Input: part model. Units: mm. Frame: model coordinates. Face numbers are marked on the shaded views. A direction names the side the tool comes from. Round coordinates to 2 decimals unless told otherwise and drop trailing zeros. Loops run counter-clockwise (first coordinate to the right, second up) from the corner with the lowest first, then second, coordinate; pieces in that order, holes last. Notation, with made-up numbers: M 35,39.25 L 94,39.25 A18 cw 94,69.25 Z; hole C -26,-19 d2. An arc over 180 degrees is marked long. Return JSON: item names as keys, results as strings. Group by question number.
1) Section D-D (y = 0.5). Output: boundary loops of the cut face in (x, z).
2) Contact query for flat-ended pins moving along their axis: P1, Ø23.5, axis at x = 0, y = 0.5, coming from the +Z side; P2, Ø14.5, axis at x = -9.5, z = 19, coming from the +Y side; P3, Ø2, axis at x = -23.5, y = -11.5, coming from the +Z side. Output: stop coordinate, or through.
3) Section A-A (z = 35). Output: boundary loops of the cut face in (x, y).
4) Material intervals for line 1 (X direction, y = -15, z = 1); line 2 (Y direction, x = 15.5, z = 1.9); line 3 (Y direction, x = 15, z = 1), sorted ascending. Write a range as from..to.
5) Section B-B (y = 16). Output: boundary loops of the cut face in (x, z), plus the area to 3 significant figures.
6) Section C-C (x = -15.5). Output: boundary loops of the cut face in (y, z).
7) Access query for the marked faces 1 and 2. Directions: +Z, -Z, +X, -X, +Y, -Y. A direction counts if a zero-diameter tool reaches every point of the face in a straight line with its end or side. Return the directions, or none.
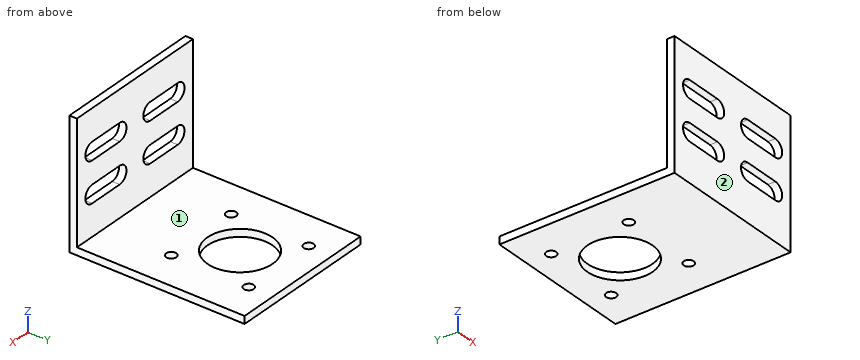
from build123d import *

# Parameters (mm, degrees)
SKETCH_1_W               = 60
SKETCH_1_H               = 70
SKETCH_1_R               = 13
EXTRUDE_1_DEPTH          = 3
SKETCH_2_W               = 60
SKETCH_2_H               = 51
EXTRUDE_2_DEPTH          = 3
SKETCH_3_R               = 2
CUT_EXTRUDE_1_DEPTH      = 10
MIRROR_3_COPY_1_SKETCH_R = 2
MIRROR_3_COPY_1_DEPTH    = 10
CUT_EXTRUDE_2_DEPTH      = 10
MIRROR_5_COPY_1_DEPTH    = 10


with BuildPart() as part:
    # 草图1 → 凸台-拉伸1 (new body)
    with BuildSketch(Plane.XY):
        with Locations((0, -9.5)):
            Rectangle(SKETCH_1_W, SKETCH_1_H)
        with Locations((0, 0.5)):
            Circle(SKETCH_1_R, mode=Mode.SUBTRACT)
    extrude(amount=EXTRUDE_1_DEPTH)

    # 草图2 → 凸台-拉伸2 (add)
    with BuildSketch(Plane.XZ.offset(44.5)):
        with Locations((0, 25.5)):
            Rectangle(SKETCH_2_W, SKETCH_2_H)
    extrude(amount=-EXTRUDE_2_DEPTH)

    # 草图3 → 切除-拉伸1 (cut)
    with BuildSketch(Plane.XY.offset(3)):
        with Locations((-15.5, 16)):
            Circle(SKETCH_3_R)
    cut_extrude_1 = extrude(amount=-CUT_EXTRUDE_1_DEPTH, mode=Mode.SUBTRACT)

    # 镜向1: 切除-拉伸1 across plane
    add(cut_extrude_1.mirror(Plane(origin=(0, 0, 0), x_dir=(0, 0, 1), z_dir=(1, 0, 0))), mode=Mode.SUBTRACT)

    # 镜向3: 切除-拉伸1 across plane
    add(cut_extrude_1.mirror(Plane.ZX.offset(0.5)), mode=Mode.SUBTRACT)

    # 镜向3 copy 1 sketch → 镜向3 copy 1 (cut)
    with BuildSketch(Plane(origin=(0, 1, 3), x_dir=(-1, 0, 0), z_dir=(0, 0, 1))):
        with Locations((-15.5, 16)):
            Circle(MIRROR_3_COPY_1_SKETCH_R)
    extrude(amount=-MIRROR_3_COPY_1_DEPTH, mode=Mode.SUBTRACT)

    # 草图4 → 切除-拉伸2 (cut)
    with BuildSketch(Plane(origin=(0, -41.5, 0), x_dir=(1, 0, 0), z_dir=(0, 1, 0))):
        with BuildLine():
            Line((-22.132037459, -15.5), (-7.867962541, -15.5))
            ThreePointArc((-7.867962541, -15.5), (-4.367962541, -19), (-7.867962541, -22.5))
            Line((-7.867962541, -22.5), (-22.132037459, -22.5))
            ThreePointArc((-22.132037459, -22.5), (-25.632037459, -19), (-22.132037459, -15.5))
        make_face()
    cut_extrude_2 = extrude(amount=-CUT_EXTRUDE_2_DEPTH, mode=Mode.SUBTRACT)

    # 镜向4: 切除-拉伸2 across plane
    add(cut_extrude_2.mirror(Plane.XY.offset(27)), mode=Mode.SUBTRACT)

    # 镜向5: 切除-拉伸2 across plane
    add(cut_extrude_2.mirror(Plane(origin=(0, 0, 0), x_dir=(0, 0, 1), z_dir=(1, 0, 0))), mode=Mode.SUBTRACT)

    # 镜向5 copy 1 sketch → 镜向5 copy 1 (cut)
    with BuildSketch(Plane(origin=(0, -41.5, 54), x_dir=(-1, 0, 0), z_dir=(0, 1, 0))):
        with BuildLine():
            Line((-22.132037459, -15.5), (-7.867962541, -15.5))
            ThreePointArc((-7.867962541, -15.5), (-4.367962541, -19), (-7.867962541, -22.5))
            Line((-7.867962541, -22.5), (-22.132037459, -22.5))
            ThreePointArc((-22.132037459, -22.5), (-25.632037459, -19), (-22.132037459, -15.5))
        make_face()
    extrude(amount=-MIRROR_5_COPY_1_DEPTH, mode=Mode.SUBTRACT)


solid = part.part
Returned:
{
 "1": {"outline": "M -30,0 L -13,0 L -13,3 L -30,3 Z; M 13,0 L 30,0 L 30,3 L 13,3 Z"},
 "2": {"P1": "passes through", "P2": "stops at y = -41.5", "P3": "stops at z = 3"},
 "3": {"outline": "M -30,-44.5 L -25.63,-44.5 L -25.63,-41.5 L -30,-41.5 Z; M -4.37,-44.5 L 4.37,-44.5 L 4.37,-41.5 L -4.37,-41.5 Z; M 25.63,-44.5 L 30,-44.5 L 30,-41.5 L 25.63,-41.5 Z"},
 "4": {"line 1": "x = -30..-17.5, -13.5..13.5, 17.5..30", "line 2": "y = -44.5..-17, -13..14, 18..25.5", "line 3": "y = -44.5..-16.94, -13.06..14.06, 17.94..25.5"},
 "5": {"outline": "M -30,0 L -17.5,0 L -17.5,3 L -30,3 Z; M -13.5,0 L 13.5,0 L 13.5,3 L -13.5,3 Z; M 17.5,0 L 30,0 L 30,3 L 17.5,3 Z", "area": "156 mm^2"},
 "6": {"outline": "M -44.5,0 L -17,0 L -17,3 L -41.5,3 L -41.5,15.5 L -44.5,15.5 Z; M -44.5,22.5 L -41.5,22.5 L -41.5,31.5 L -44.5,31.5 Z; M -44.5,38.5 L -41.5,38.5 L -41.5,51 L -44.5,51 Z; M -13,0 L 14,0 L 14,3 L -13,3 Z; M 18,0 L 25.5,0 L 25.5,3 L 18,3 Z"},
 "7": {"face 1": "+Z, +X, -X, +Y", "face 2": "+Z, -Z, +X, -X, -Y"}
}
